Source: three-view drawing plus pictorial views. Frame: mm from the lowest corner of the part. Give positions to 0.01 mm unless a question says otherwise; leave off trailing zeros. Order: outer loops, then holes, each group sorted by start corner. A loop starts at its lowest first (then second) coordinate and runs counter-clockwise, first axis right, second up. Notation, with made-up numbers: (-40, -39) - (-27, -39) arc R35 cw to (-27, -6) - close; hole circle Ø6 at (0.25, -21.5). An arc over 180 degrees is marked (long way). Answer in a Markdown table with one row per item. Add a question column.
1. Contact query for a flat-ended pin moving along its axis: pin 1 (10 mm diameter, centred on x = 295, z = 17, fed in from -Y). Output: stop coordinate, or through.
2. Ray query, line 1 (X direction, y = 304.8, z = 5); line 2 (X direction, y = 196, z = 13.75); line 3 (Y direction, x = 38.1, z = 8.25). Return the intervals inside material, ascending. Write a range as [from, to].
3. Section query A-A on y = 86. Return loops of the section in (x, z).
4. Section query C-C on x = 285.5. Return loops of the section in (y, z), and give its area (3 significant figures).
5. Section query B-B on z = 14. Return loops of the section in (x, y).
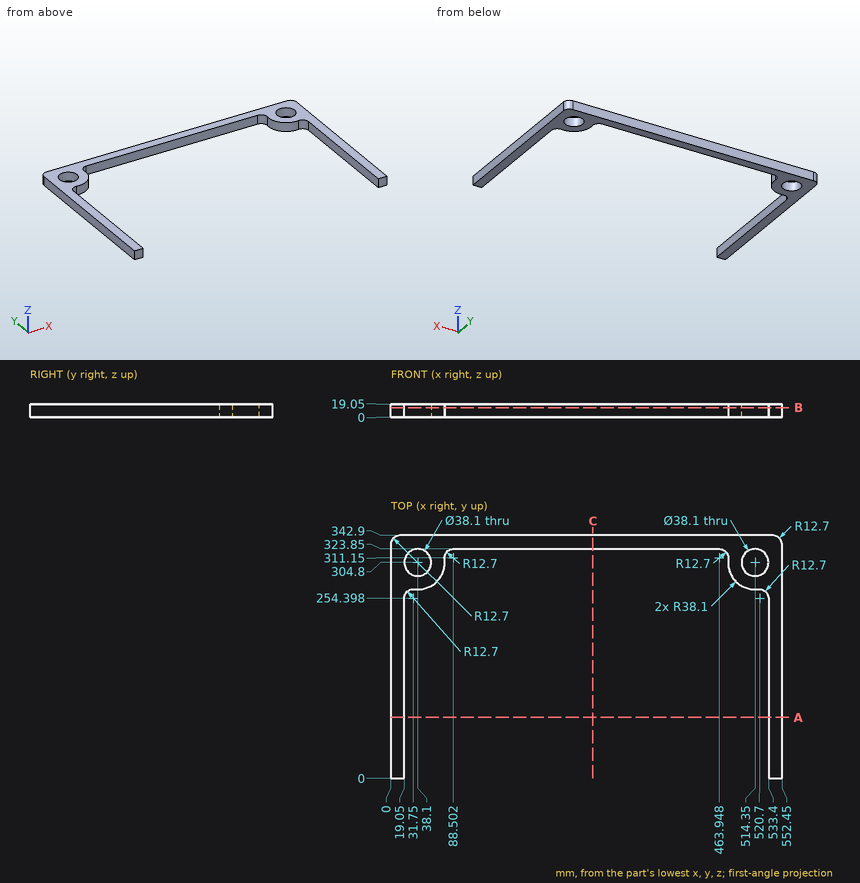
Answer:
| question | item | result |
|---|---|---|
| 1 | pin 1 | stops at y = 323.85 |
| 2 | line 1 | x = [0, 19.05], [57.15, 76.2], [476.25, 495.3], [533.4, 552.45] |
| 2 | line 2 | x = [0, 19.05], [533.4, 552.45] |
| 2 | line 3 | y = [266.7, 285.75], [323.85, 342.9] |
| 3 | outline | (0, 0) - (19.05, 0) - (19.05, 19.05) - (0, 19.05) - close; (533.4, 0) - (552.45, 0) - (552.45, 19.05) - (533.4, 19.05) - close |
| 4 | outline | (323.85, 0) - (342.9, 0) - (342.9, 19.05) - (323.85, 19.05) - close |
| 4 | area | 363 mm² |
| 5 | outline | (0, 0) - (19.05, 0) - (19.05, 254.4) arc R12.7 cw to (33.34, 267) arc R38.1 ccw to (75.9, 309.56) arc R12.7 cw to (88.5, 323.85) - (463.95, 323.85) arc R12.7 cw to (476.55, 309.56) arc R38.1 ccw to (519.11, 267) arc R12.7 cw to (533.4, 254.4) - (533.4, 0) - (552.45, 0) - (552.45, 330.2) arc R12.7 ccw to (539.75, 342.9) - (12.7, 342.9) arc R12.7 ccw to (0, 330.2) - close; hole circle Ø38.1 at (38.1, 304.8); hole circle Ø38.1 at (514.35, 304.8) |
